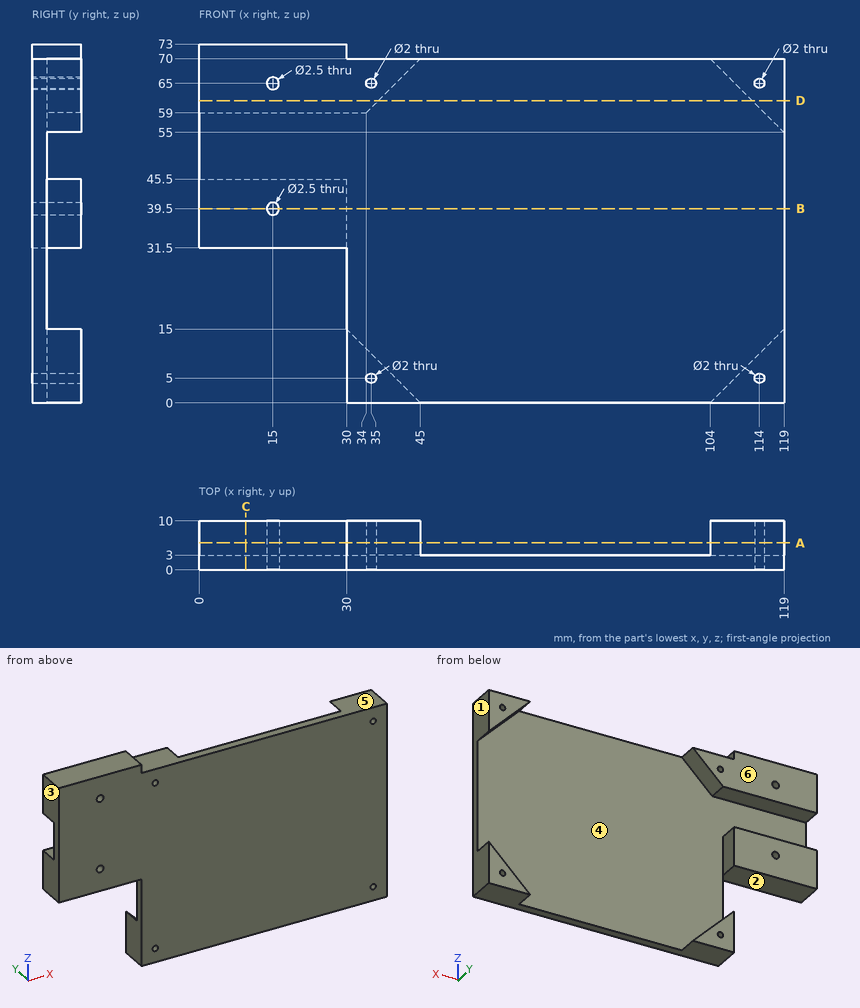
Here's the drawing with two shaded views (mm, measured from the low corner). I have some questions. A direction names the side the tool comes from. Coordinates: 2 decimals unless noted, no trailing zeros. Order: outer loops, then holes, each group sorted by start corner. A loop starts at its lowest first (then second) coordinate and runs counter-clockwise, first axis right, second up. Notation, with made-up numbers: (-5.5, 52) - (53.5, 52) arc R24 ccw to (53.5, 82) - close; hole circle Ø6 at (-5, 34). An arc over 180 degrees is marked (long way). Answer in a Markdown table with one row per item.
1. Suppose I cut it at B-B (z = 39.5). Please give me the cut outline in (x, y).
Reply:
| item | result |
|---|---|
| outline | (0, 0) - (13.75, 0) - (13.75, 10) - (0, 10) - close; (16.25, 0) - (119, 0) - (119, 3) - (30, 3) - (30, 10) - (16.25, 10) - close |
2. For pin 1 (8 mm diameter, centred on x = 52.5, z = 20, fed in from +Y); pin 2 (3 mm diameter, centred on x = 12.5, y = 3, fed in from -Z); pin 3 (6 mm diameter, centred on y = 3, z = 8.5, fed in from -X); pin 4 (1 mm diameter, centred on x = 57.5, y = 2.5, fed in from -Z), each with a flat end and sliding along its axis, tell me the tip position at first contact or that it passes through.
Reply:
| item | result |
|---|---|
| pin 1 | stops at y = 3 |
| pin 2 | stops at z = 31.5 |
| pin 3 | stops at x = 30 |
| pin 4 | stops at z = 0 |
3. Suppose I cut it at C-C (x = 9.5). Please give me the cut outline in (y, z).
Reply:
| item | result |
|---|---|
| outline | (0, 31.5) - (10, 31.5) - (10, 45.5) - (3, 45.5) - (3, 59) - (10, 59) - (10, 73) - (0, 73) - close |
4. If we mould it in two halves opening along X, with no side actions, what happens to the marked faces 1, 2, 3 and 4? For each: pulls with the +X half, pulls with the -X half, needs draft (parallel to the pull), parting line crosses it, or undercut.
Reply:
| item | result |
|---|---|
| face 1 | pulls with the +X half |
| face 2 | needs draft |
| face 3 | pulls with the -X half |
| face 4 | undercut |
5. Suppose I cut it at A-A (y = 5.5). Give the number of separate pieces and of enclosed holes in the cut face, and give its area (3 significant figures).
Reply:
| item | result |
|---|---|
| separate pieces | 5 |
| enclosed holes | 6 |
| area | 1,260 mm^2 |
6. If I drill on line 1 along X through (y, z) = (5.75, 5); line 2 along X through (y, z) = (7, 65); line 3 along X through (y, z) = (2.75, 5), over which ranges is the centre line in solid material (lowest first)?
Reply:
| item | result |
|---|---|
| line 1 | x = 30 to 34, 36 to 40, 109 to 113, 115 to 119 |
| line 2 | x = 0 to 13.75, 16.25 to 34, 36 to 40, 109 to 113, 115 to 119 |
| line 3 | x = 30 to 34, 36 to 113, 115 to 119 |
7. Suppose I cut it at D-D (z = 61.5). Please give me the cut outline in (x, y).
Reply:
| item | result |
|---|---|
| outline | (0, 0) - (119, 0) - (119, 10) - (112.5, 10) - (112.5, 3) - (36.5, 3) - (36.5, 10) - (0, 10) - close |
8. For the marked faces 5 and 6, which set-ups out of +Z, -Z, +X, -X, +Y, -Y let a thin tool reach every point of the face, with its end or its side?
Reply:
| item | result |
|---|---|
| face 5 | +Z, +X, +Y, -Y |
| face 6 | +Z, -Z, +X, -X, +Y |
